Can you work these out from the model? Positions are in its coordinate system, mm. A direction names the side the tool comes from. Round coordinates to 2 decimals unless told otherwise and drop trailing zeros. Loops run counter-clockwise (first coordinate to the right, second up) from the corner with the lowest first, then second, coordinate; pieces in that order, holes last. Notation, with made-up numbers: M 23,79 L 59,79 A32 ccw 59,105 Z; hole C 56,41.5 d7. An arc over 180 degrees is marked long. Return JSON: item names as keys, results as strings.
```python
from build123d import *

# Parameters (mm, degrees)
FILLET1_R           = 0.5
BOSS_EXTRUDE1_REACH = 62.882
BOSS_EXTRUDE1_START = 14
SKETCH2_W           = 0.7
SKETCH2_H           = 1
CIRPATTERN1_COUNT   = 4


with BuildPart() as part:
    # Sketch1 → Revolve1 (revolve)
    with BuildSketch(Plane(origin=(0, 0, 0), x_dir=(0, 0, -1), z_dir=(1, 0, 0))):
        Polygon((3.15, 33), (3.15, 6.8), (3.5, 6.8), (3.5, 0), (4.5, 0), (4.5, 6.8), (5.4, 6.8), (5.4, 5.8), (6.4, 5.8), (6.4, 7.8), (4.8, 7.8), (4.8, 35.5), (3.95, 35.5), (3.95, 42.8), (4.15, 43.146410162), (4.15, 44.5), (3.95, 44.5), (3.95, 46), (2.9, 46), (2.9, 37.5), (1.75, 34), (1.75, 33), align=None)
    revolve(axis=Axis((0, 0, 0), (0, 1, 0)))

    # Fillet1
    fillet1_edges = [part.edges().sort_by_distance(p)[0] for p in [
        (0, 7.8, 6.4),
    ]]
    fillet(fillet1_edges, radius=FILLET1_R)

    # Sketch2 → Boss-Extrude1 (add, up to next)
    with BuildSketch(Plane(origin=(0, 0, 0), x_dir=(-1, 0, 0), z_dir=(0, 1, 0)).offset(BOSS_EXTRUDE1_START), mode=Mode.PRIVATE) as boss_extrude1_sk1:
        with Locations((0, 2.65)):
            Rectangle(SKETCH2_W, SKETCH2_H)
    boss_extrude1_tool1 = extrude(boss_extrude1_sk1.sketch, amount=BOSS_EXTRUDE1_REACH, mode=Mode.PRIVATE) - part.part
    boss_extrude1 = boss_extrude1_tool1.solids().sort_by_distance((0, 14, 2.65))[0]
    add(boss_extrude1)

    # CirPattern1: Boss-Extrude1 ×4 about axis
    cirpattern1_axis = Axis((0, 0, 0), (0, 1, 0))
    for i in range(1, CIRPATTERN1_COUNT):
        add(boss_extrude1.rotate(cirpattern1_axis, i * 360 / CIRPATTERN1_COUNT))


solid = part.part
```
Q1. On a 3-axis mill with a long thin cutter (end or side, diameter ignored), from which of +Z, -Z, +X, -X, +Y, -Y can I reach the whole of each face in a straight line? I mean faces 1 (the cylindrical face through (4.05, 43.83, 0.9)), 2 (the flat face through (-0.35, 23.4, 2.6)), 3 (the flat face through (-3, 46, 1)). Say none if no direction works.
Results:
{"face 1": "+Y", "face 2": "-Y", "face 3": "+Z, -Z, +X, -X, +Y"}
Q2. If I drill on line 1 along X through (y, z) = (6.25, 0); line 2 along X through (y, z) = (12.75, 0); line 3 along Z through (x, y) = (0, 16.25), over which ranges is the centre line in solid material (lowest first)?
Results:
{"line 1": "x = -6.4 to -5.4, -4.5 to -3.5, 3.5 to 4.5, 5.4 to 6.4", "line 2": "x = -4.8 to -3.15, 3.15 to 4.8", "line 3": "z = -4.8 to -2.15, 2.15 to 4.8"}
Q3. Suppose I cut it at A-A, the plane y = 16.5. Please give me the cut outline in (x, z).
Results:
{"outline": "C 0,0 d9.6; hole M -3.13,-0.35 A3.15 ccw -0.35,-3.13 L -0.35,-2.15 L 0.35,-2.15 L 0.35,-3.13 A3.15 ccw 3.13,-0.35 L 2.15,-0.35 L 2.15,0.35 L 3.13,0.35 A3.15 ccw 0.35,3.13 L 0.35,2.15 L -0.35,2.15 L -0.35,3.13 A3.15 ccw -3.13,0.35 L -2.15,0.35 L -2.15,-0.35 Z"}
Q4. Thinking about a two-plate mould opening in X: for faces 4 (the flat face through (-4, 6.8, -3)), 5 (the cylindrical face through (0.67, 33.493, -1.617)), 6 (the flat face through (5, 5.8, -3)), 7 (the cylindrical face through (-4.05, 21.84, -2.58)), which applies, pulls with the +X half, pulls with the -X half, needs draft (parallel to the pull), parting line crosses it, or undercut?
Results:
{"face 4": "undercut", "face 5": "undercut", "face 6": "needs draft", "face 7": "parting line crosses it"}
Q5. Suppose I cut it at B-B, the plane y = 5. Please give me the cut outline in (x, z).
Results:
{"outline": "C 0,0 d9; hole C 0,0 d7"}
Q6. I'm going to push flat-ended pins straight in: pin 1 Ø4 at (y, z) = (9, -1.5) entering from -X; pin 2 Ø4 at (x, z) = (0, 0) entering from -Y; pin 3 Ø0.8 at (x, y) = (2.5, 27) entering from -Z. Where does each tip first touch, or does it pass through?
Results:
{"pin 1": "stops at x = -6.39", "pin 2": "stops at y = 33", "pin 3": "stops at z = -4.32"}
